Work out the finished part from the listing and answer in its coordinate system (mm). A direction names the side the tool comes from. Coordinates: 2 decimals unless noted, no trailing zeros. Loops run counter-clockwise (first coordinate to the right, second up) from the corner with the lowest first, then second, coordinate; pieces in that order, holes last. Notation, with made-up numbers: (61.5, -13) -> (65.5, -13) arc R27 cw to (65.5, 20) -> close; hole circle Ø5 at (-28, 81.5). An arc over 180 degrees is marked (long way). Use a Markdown table: item, result.
from build123d import *

# Parameters (mm, degrees)
SKETCH1_W           = 20.35
SKETCH1_H           = 15.24
SKETCH1_R           = 1.5
BOSS_EXTRUDE1_DEPTH = 1.6
SKETCH2_W           = 5
SKETCH2_H           = 3
SKETCH2_W_2         = 3
SKETCH2_H_2         = 2.5
SKETCH2_H_3         = 1.7
SKETCH2_W_3         = 1
SKETCH2_H_4         = 2
SKETCH2_W_4         = 0.6
BOSS_EXTRUDE2_DEPTH = 1.5
SKETCH3_R           = 0.5
CUT_EXTRUDE1_DEPTH  = 2.6
LPATTERN1_COUNT     = 5
LPATTERN1_PITCH     = 2.54
LPATTERN1_COL_COUNT = 4
LPATTERN1_COL_PITCH = 2.54


with BuildPart() as part:
    # Sketch1 → Boss-Extrude1 (new body)
    with BuildSketch(Plane.XY):
        Rectangle(SKETCH1_W, SKETCH1_H)
        with Locations((-7.375, 4.62)):
            Circle(SKETCH1_R, mode=Mode.SUBTRACT)
        with Locations((7.375, 4.62)):
            Circle(SKETCH1_R, mode=Mode.SUBTRACT)
    extrude(amount=BOSS_EXTRUDE1_DEPTH)

    # Sketch2 → Boss-Extrude2 (add)
    with BuildSketch(Plane.XY.offset(1.6)):
        with Locations((0, 1.12)):
            Rectangle(SKETCH2_W, SKETCH2_H)
        with Locations((-8.175, 0.37)):
            Rectangle(SKETCH2_W_2, SKETCH2_H_2)
        with Locations((0, 4.77)):
            Rectangle(SKETCH2_W_2, SKETCH2_H_3)
        with Locations((3.875, 4.62)):
            Rectangle(SKETCH2_W_3, SKETCH2_H_4)
        with Locations((-3.875, 4.62)):
            Rectangle(SKETCH2_W_3, SKETCH2_H_4)
        with Locations((4.475, 0.38)):
            Rectangle(SKETCH2_W_4, SKETCH2_H_4)
        with Locations((5.575, 0.38)):
            Rectangle(SKETCH2_W_4, SKETCH2_H_4)
        with Locations((6.675, 0.38)):
            Rectangle(SKETCH2_W_4, SKETCH2_H_4)
    extrude(amount=BOSS_EXTRUDE2_DEPTH)

    # Sketch3 → Cut-Extrude1 (cut, through all)
    with BuildSketch(Plane.XY.offset(1.6)):
        with Locations((-1.28, -6.62)):
            Circle(SKETCH3_R)
    cut_extrude1 = extrude(amount=-CUT_EXTRUDE1_DEPTH, mode=Mode.SUBTRACT)

    # LPattern1: Cut-Extrude1 ×5
    with Locations(*[(i * LPATTERN1_PITCH, 0, 0) for i in range(1, LPATTERN1_COUNT)]):
        add(cut_extrude1, mode=Mode.SUBTRACT)

    # LPattern1 col: Cut-Extrude1 ×4
    with Locations(*[(-i * LPATTERN1_COL_PITCH, 0, 0) for i in range(1, LPATTERN1_COL_COUNT)]):
        add(cut_extrude1, mode=Mode.SUBTRACT)


solid = part.part
Q1. Given pin 1 Ø1.6 at (x, z) = (0, 2.5) entering from +Y; pin 2 Ø1.6 at (y, z) = (0, 2.5) entering from -X (3 decimals); pin 3 Ø5 at (x, y) = (7.375, 4.62) entering from +Z, each flat-ended and moving along its own axis, determine where each tip first touches the part or whether it passes through.
Solved:
| item | result |
|---|---|
| pin 1 | y = 5.62 |
| pin 2 | x = -9.675 |
| pin 3 | z = 1.6 |
Q2. For faces 5 (the flat face through (-8, 1.62, 2)), 6 (the flat face through (0, -0.38, 2)), 7 (the flat face through (4, 3.62, 2)), determine the directions among +Z, -Z, +X, -X, +Y, -Y from which every point of the face is accessible in a straight line to the end or side of a thin tool.
Solved:
| item | result |
|---|---|
| face 5 | +Z, -X, +Y |
| face 6 | +Z, -Y |
| face 7 | +Z, +X, -X |
Q3. Determine the mould class of faces 1 (the flat face through (0, -7.62, 1)), 2 (the cylindrical face through (6.571, -7.064, 0.811)), 3 (the flat face through (4, 5.62, 2)), 4 (the flat face through (3.375, 5, 2)) for opening direction Y: pulls with the +Y half, pulls with the -Y half, needs draft (parallel to the pull), parting line crosses it, or undercut.
Solved:
| item | result |
|---|---|
| face 1 | pulls with the -Y half |
| face 2 | undercut |
| face 3 | pulls with the +Y half |
| face 4 | needs draft |
Q4. Section C-C on x = -6.36 is taken. Determine the outline of the cut face in (y, z), and give its area (3 significant figures).
Solved:
| item | result |
|---|---|
| outline | (-7.62, 0) -> (-7.12, 0) -> (-7.12, 1.6) -> (-7.62, 1.6) -> close; (-6.12, 0) -> (3.52, 0) -> (3.52, 1.6) -> (-6.12, 1.6) -> close; (5.72, 0) -> (7.62, 0) -> (7.62, 1.6) -> (5.72, 1.6) -> close |
| area | 19.2 mm² |
Q5. Section B-B on x = -3.82 is taken. Determine the outline of the cut face in (y, z), and give its area (3 significant figures).
Solved:
| item | result |
|---|---|
| outline | (-7.62, 0) -> (-7.12, 0) -> (-7.12, 1.6) -> (-7.62, 1.6) -> close; (-6.12, 0) -> (7.62, 0) -> (7.62, 1.6) -> (5.62, 1.6) -> (5.62, 3.1) -> (3.62, 3.1) -> (3.62, 1.6) -> (-6.12, 1.6) -> close |
| area | 25.8 mm² |
Q6. Section A-A on z = 1.9 is taken. State how many separate pieces and enclosed holes the cut face has, and give its area (3 significant figures).
Solved:
| item | result |
|---|---|
| separate pieces | 8 |
| enclosed holes | 0 |
| area | 35.2 mm² |
Q7. Consider line 1 (X direction, y = 0.5, z = 1.9) (3 decimals); line 2 (X direction, y = 4, z = 2.3) (3 decimals); line 3 (Y direction, x = 7.25, z = 0.5). Determine where each line is inside the solid, lowest interval first. Write a range as [from, to].
Solved:
| item | result |
|---|---|
| line 1 | [-9.675, -6.675], [-2.5, 2.5], [4.175, 4.775], [5.275, 5.875], [6.375, 6.975] |
| line 2 | [-4.375, -3.375], [-1.5, 1.5], [3.375, 4.375] |
| line 3 | [-7.62, 3.13], [6.11, 7.62] |
